The listing builds one solid part. Answer for the finished solid, in the listing's coordinates (mm). Face numbers are marked on the shaded views. A direction names the side the tool comes from. Coordinates: 2 decimals unless noted, no trailing zeros. Order: outer loops, then holes, each group sorted by start corner. A loop starts at its lowest first (then second) coordinate and runs counter-clockwise, first axis right, second up. Notation, with made-up numbers: (34, 27.5) -> (40, 27.5) arc R24 cw to (40, 58.5) -> close; hole circle Ø3 at (84.25, 65.5). An arc over 180 degrees is marked (long way). Answer in a Markdown table with one row per item.
```python
from build123d import *

# Parameters (mm, degrees)
F1_DEPTH = 76.2
F2_R     = 9.525
F3_DEPTH = 25.4
F4_R     = 9.525


with BuildPart() as f1:
    # F0 (on Top) → F1 (new body)
    with BuildSketch(Plane.XY):
        with BuildLine():
            Line((-41.285193, 12.7), (-41.285193, 31.75))
            Line((-41.285193, 31.75), (-53.985193, 31.75))
            Line((-53.985193, 31.75), (-53.985193, 9.525))
            ThreePointArc((-53.985193, 9.525), (-51.195385, 2.789808), (-44.460193, 0))
            Line((-44.460193, 0), (0.789147, 0))
            ThreePointArc((0.789147, 0), (6.937508, -2.250161), (10.180923, -7.9375))
            ThreePointArc((10.180923, -7.9375), (57.139807, -47.625), (104.09869, -7.9375))
            ThreePointArc((104.09869, -7.9375), (107.342106, -2.250161), (113.490467, 0))
            Line((113.490467, 0), (158.739807, 0))
            ThreePointArc((158.739807, 0), (165.474999, 2.789808), (168.264807, 9.525))
            Line((168.264807, 9.525), (168.264807, 31.75))
            Line((168.264807, 31.75), (155.564807, 31.75))
            Line((155.564807, 31.75), (155.564807, 12.7))
            Line((155.564807, 12.7), (89.673875, 12.7))
            ThreePointArc((89.673875, 12.7), (57.139807, -34.925), (24.605738, 12.7))
            Line((24.605738, 12.7), (-41.285193, 12.7))
        make_face()
    extrude(amount=F1_DEPTH)

    # F2 (on face) → F3 (cut)
    with BuildSketch(Plane.XZ):
        with Locations((136.115137, 38.1)):
            Circle(F2_R)
        with Locations((-22.6314, 38.1)):
            Circle(F2_R)
    extrude(amount=-F3_DEPTH, mode=Mode.SUBTRACT)

    # F4
    f4_edges = [f1.edges().sort_by_distance(p)[0] for p in [
        (-47.635193, 31.75, 76.2),
        (-47.635193, 31.75, 0),
        (161.914807, 31.75, 0),
        (161.914807, 31.75, 76.2),
    ]]
    fillet(f4_edges, radius=F4_R)


solid = f1.part
```
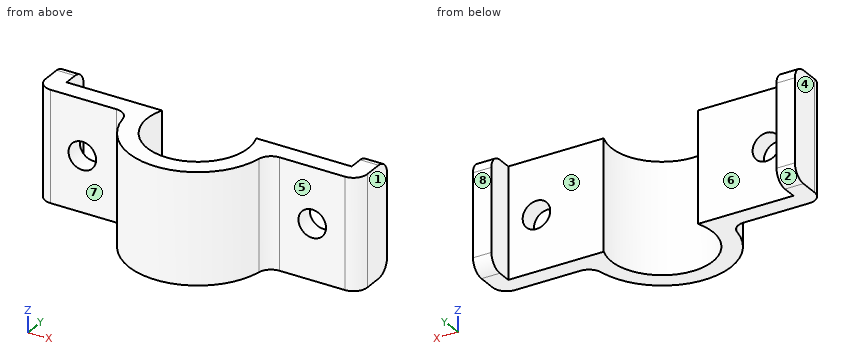
(1) Flat-ended cylindrical pins translate along their axes: pin 1 (1 mm diameter, centred on y = 2.5, z = 34.5, fed in from -X); pin 2 (3 mm diameter, centred on y = -38, z = 26.5, fed in from +X); pin 3 (2 mm diameter, centred on x = 51, z = 11.5, fed in from -Y). Find the tip coordinate at first contact, or state that the pin passes through.
Check values:
| item | result |
|---|---|
| pin 1 | x = -51.4 |
| pin 2 | x = 87.73 |
| pin 3 | y = -47.35 |
(2) For a pull along X with two mould halves and no side action, classify the marked faces 1, 2 and 3 as released by +X, released by -X, zero draft, split by the parting line, or undercut.
Check values:
| item | result |
|---|---|
| face 1 | released by +X |
| face 2 | zero draft |
| face 3 | undercut |
(3) Which of the six approach directions +Z, -Z, +X, -X, +Y, -Y give full straight-line access (tool end or side, diameter ignored) to the marked faces 4, 5, 6, 7 and 8?
Check values:
| item | result |
|---|---|
| face 4 | +Z, -Z, -X, +Y, -Y |
| face 5 | +Z, -Z, +X, -Y |
| face 6 | +Z, -Z, +Y |
| face 7 | +Z, -Z, -X, -Y |
| face 8 | +Z, -Z, +X, -X, +Y |
(4) Find the intervals of material crossed by line 1 along X through (y, z) = (4.5, 39.5); line 2 along Y through (x, z) = (134, 17); line 3 along X through (y, z) = (3, 38), in increasing order. Write a range as from..to.
Check values:
| item | result |
|---|---|
| line 1 | -52.55..-32.05, -13.21..22.51, 91.77..126.69, 145.54..166.83 |
| line 2 | 0..12.7 |
| line 3 | -51.4..-32.16, -13.11..22.34, 91.94..126.59, 145.64..165.68 |
(5) A cutting plane is placed at A-A, the plane z = 38.1. Count the separate pieces of the cut face and the enclosed holes in it, then the cut area to 3 significant figures.
Check values:
| item | result |
|---|---|
| separate pieces | 3 |
| enclosed holes | 0 |
| area | 3,590 mm² |
(6) A cutting plane is placed at C-C, the plane x = 86.5. Determine the outline of the cut face in (y, z).
Check values:
| item | result |
|---|---|
| outline | (-37.5, 0) -> (-18.91, 0) -> (-18.91, 76.2) -> (-37.5, 76.2) -> close |
